from build123d import *

# Parameters (mm, degrees)
SKETCH2_R          = 5
CUT_EXTRUDE1_DEPTH = 44
CHAMFER1_SIZE      = 0.5


with BuildPart() as part:
    # Sketch1 → Revolve1 (revolve)
    with BuildSketch(Plane.XY):
        Polygon((-2.846534653, 10), (9.653465347, 10), (9.653465347, 0), (7.153465347, 0), (7.153465347, -33), (-2.846534653, -33), align=None)
    revolve(axis=Axis((-2.846534653, -33, 0), (0, 1, 0)))

    # Sketch2 → Cut-Extrude1 (cut, through all)
    with BuildSketch(Plane(origin=(0, 10, 0), x_dir=(1, 0, 0), z_dir=(0, 1, 0))):
        with Locations((-2.846534653, 0)):
            Circle(SKETCH2_R)
    extrude(amount=-CUT_EXTRUDE1_DEPTH, mode=Mode.SUBTRACT)

    # Chamfer1
    chamfer1_edges = [part.edges().sort_by_distance(p)[0] for p in [
        (-12.846534653, -33, 0),
        (-15.346534653, 0, 0),
        (-15.346534653, 10, 0),
    ]]
    chamfer(chamfer1_edges, length=CHAMFER1_SIZE)


solid = part.part
CAD build for the part. Positions are in the model's coordinates, mm. Give positions to 0.01 mm unless a question says otherwise; leave off trailing zeros. Loops run counter-clockwise (first coordinate to the right, second up) from the corner with the lowest first, then second, coordinate; pieces in that order, holes last. Notation, with made-up numbers: M 75.5,-30.5 L 126.5,-30.5 A21 cw 126.5,-10.5 Z; hole C 76.5,74.25 d7. An arc over 180 degrees is marked long. Answer in a Markdown table with one row per item. Add a question column.
Item 1: Band-saw the part on B-B on y = 7.5. Give the cut face in (x, z), then the cut area to 3 significant figures.
Item 2: Mould opens along Z. For faces 1 (the face through (-6, 0, -10)), 2 (the face through (-7.84, -11.2, -0.22)), 3 (the face through (-10.782, -16.478, 6.085)) say: +Z half, -Z half, draft (parallel to the pull), parting line (faces both ways), or undercut.
Item 3: Probe probe 1 along X at (y, z) = (2, 0.25); probe 2 along X at (y, z) = (-20, 0); probe 3 along Z at (x, y) = (-1.75, -12.5). List the from-to ranges inside material, lowest first.
Item 4: Band-saw the part on C-C on y = -8. Give the cut face in (x, z), then the cut area to 3 significant figures.
Item 5: Drop flat-ended pins along their axis: P1, Ø3, axis at x = 5, y = -25.5, coming from the +Z side; P2, Ø6, axis at x = -2.85, z = 0, coming from the +Y side; P3, Ø12, axis at x = 7, y = -10, coming from the +Z side; P4, Ø8, axis at x = -11, y = -14, coming from the -Z side. Give the stop position or say it passes through.
Item 6: Band-saw the part on A-A on z = 0. Give the cut face in (x, y), then the cut area to 3 significant figures.
Reply:
| question | item | result |
|---|---|---|
| 1 | outline | C -2.85,0 d25; hole C -2.85,0 d10 |
| 1 | area | 412 mm^2 |
| 2 | face 1 | draft |
| 2 | face 2 | undercut |
| 2 | face 3 | parting line |
| 3 | probe 1 | x = -15.34 to -7.84, 2.15 to 9.65 |
| 3 | probe 2 | x = -12.85 to -7.85, 2.15 to 7.15 |
| 3 | probe 3 | z = -9.94 to -4.88, 4.88 to 9.94 |
| 4 | outline | C -2.85,0 d20; hole C -2.85,0 d10 |
| 4 | area | 236 mm^2 |
| 5 | P1 | stops at z = 7.73 |
| 5 | P2 | passes through |
| 5 | P3 | stops at z = 9.23 |
| 5 | P4 | stops at z = -9.1 |
| 6 | outline | M -15.35,0.5 L -14.85,0 L -12.85,0 L -12.85,-32.5 L -12.35,-33 L -7.85,-33 L -7.85,10 L -14.85,10 L -15.35,9.5 Z; M 2.15,-33 L 6.65,-33 L 7.15,-32.5 L 7.15,0 L 9.15,0 L 9.65,0.5 L 9.65,9.5 L 9.15,10 L 2.15,10 Z |
| 6 | area | 479 mm^2 |
